```python
from build123d import *

# Parameters (mm, degrees)
SKETCH1_W                 = 3
SKETCH1_H                 = 15
BOSS_EXTRUDE1_START       = 9
SKETCH2_R                 = 5
BOSS_EXTRUDE1_DEPTH       = 9
M5X0_8_TAPPED_HOLE1_D     = 4.2
M5X0_8_TAPPED_HOLE1_DEPTH = 12.4
M5X0_8_TAPPED_HOLE1_TIP   = 1.2618073


with BuildPart() as part:
    # Sketch1 → Revolve1 (revolve)
    with BuildSketch(Plane.XY, mode=Mode.PRIVATE) as revolve1_sk:
        with Locations((-6.5, -4.132653061)):
            Rectangle(SKETCH1_W, SKETCH1_H)
    revolve(revolve1_sk.sketch.rotate(Axis((0, 8.367346939, 0), (0, -1, 0)), 270), axis=Axis((0, 8.367346939, 0), (0, -1, 0)))

    # Sketch2 → Boss-Extrude1 (add)
    with BuildSketch(Plane(origin=(0, 3.367346939, 0), x_dir=(1, 0, 0), z_dir=(0, 1, 0)).offset(BOSS_EXTRUDE1_START)):
        with BuildLine():
            Line((-6.5, 11.258330249), (-18.5, 4.330127019))
            ThreePointArc((-18.5, 4.330127019), (-21, 0), (-18.5, -4.330127019))
            Line((-18.5, -4.330127019), (-6.5, -11.258330249))
            ThreePointArc((-6.5, -11.258330249), (0, -13), (6.5, -11.258330249))
            Line((6.5, -11.258330249), (18.5, -4.330127019))
            ThreePointArc((18.5, -4.330127019), (21, 0), (18.5, 4.330127019))
            Line((18.5, 4.330127019), (6.5, 11.258330249))
            ThreePointArc((6.5, 11.258330249), (0, 13), (-6.5, 11.258330249))
        make_face()
        with Locations(Location((0, 0, 0), (0, 0, 270))):
            Circle(SKETCH2_R, mode=Mode.SUBTRACT)
    extrude(amount=-BOSS_EXTRUDE1_DEPTH)

    # M5x0.8 Tapped Hole1
    with Locations(Plane(origin=(-16, 12.367346939, 0), x_dir=(0, 0, 1), z_dir=(0, 1, 0))):
        with Locations((0, 0), (0, 32)):
            Hole(M5X0_8_TAPPED_HOLE1_D / 2, depth=M5X0_8_TAPPED_HOLE1_DEPTH)
            with Locations((0, 0, -(M5X0_8_TAPPED_HOLE1_DEPTH + M5X0_8_TAPPED_HOLE1_TIP / 2))):  # 118° drill point
                Cone(0, M5X0_8_TAPPED_HOLE1_D / 2, M5X0_8_TAPPED_HOLE1_TIP, mode=Mode.SUBTRACT)


solid = part.part
```
Geometry: final body of the model. Coordinates: model frame, mm. A direction names the side the tool comes from. Give positions to 0.01 mm unless a question says otherwise; leave off trailing zeros. Loops run counter-clockwise (first coordinate to the right, second up) from the corner with the lowest first, then second, coordinate; pieces in that order, holes last. Notation, with made-up numbers: (53.5, 5) -> (98.5, 5) arc R15 cw to (98.5, 12) -> close; hole circle Ø2 at (5.25, -10.5). An arc over 180 degrees is marked (long way). Return JSON: item names as keys, results as strings.
Item 1: Section B-B, the plane z = 0. Output: boundary loops of the cut face in (x, y).
Filled in:
{"outline": "(-21, 3.37) -> (-18.1, 3.37) -> (-18.1, 12.37) -> (-21, 12.37) -> close; (-13.9, 3.37) -> (-8, 3.37) -> (-8, -11.63) -> (-5, -11.63) -> (-5, 12.37) -> (-13.9, 12.37) -> close; (5, -11.63) -> (8, -11.63) -> (8, 3.37) -> (13.9, 3.37) -> (13.9, 12.37) -> (5, 12.37) -> close; (18.1, 3.37) -> (21, 3.37) -> (21, 12.37) -> (18.1, 12.37) -> close"}
Item 2: Section D-D, the plane z = -3.25. Output: boundary loops of the cut face in (x, y), plus the area to 3 significant figures.
Filled in:
{"outline": "(-19.8, 3.37) -> (-7.31, 3.37) -> (-7.31, -11.63) -> (-3.8, -11.63) -> (-3.8, 12.37) -> (-19.8, 12.37) -> close; (3.8, -11.63) -> (7.31, -11.63) -> (7.31, 3.37) -> (19.8, 3.37) -> (19.8, 12.37) -> (3.8, 12.37) -> close", "area": "393 mm^2"}
Item 3: Line query: line 1 (Z direction, x = 0, y = 6.25); line 2 (X direction, y = -7, z = 0); line 3 (Y direction, x = 12, z = 4). Output: solid intervals per line, ascending.
Filled in:
{"line 1": "-13 to -5, 5 to 13", "line 2": "-8 to -5, 5 to 8", "line 3": "3.37 to 12.37"}
Item 4: Mould query, pull axis X, two halves, no side actions, for faces 1 (the cylindrical face through (21, 8, 0)), 2 (the flat face through (5.2, -11.633, -0.1)), 3 (the cylindrical face through (17.77, 7.8, -1.13)), 4 (the cylindrical face through (-13.918, 7.804, 0.273)). Classes: released by +X, released by -X, zero draft, split by the parting line, or undercut.
Filled in:
{"face 1": "released by +X", "face 2": "zero draft", "face 3": "undercut", "face 4": "undercut"}
Item 5: Pin query (flat end, axial travel): P1, Ø10, axis at x = -16.5, y = 1.5, coming from the +Z side; P2, Ø3, axis at x = -6.5, y = 8.5, coming from the +Z side; P3, Ø6, axis at x = -6, y = 9.5, coming from the +Z side. Return the tip coordinate at first contact, or that it passes through.
Filled in:
{"P1": "z = 8.16", "P2": "z = 12", "P3": "z = 12.65"}
Item 6: Section A-A, the plane x = 0. Output: boundary loops of the cut face in (y, z).
Filled in:
{"outline": "(-11.63, -8) -> (3.37, -8) -> (3.37, -13) -> (12.37, -13) -> (12.37, -5) -> (-11.63, -5) -> close; (-11.63, 5) -> (12.37, 5) -> (12.37, 13) -> (3.37, 13) -> (3.37, 8) -> (-11.63, 8) -> close"}
Item 7: Access query for faces 5 (the cylindrical face through (0, 8, -13)), 6 (the flat face through (0, 3.367, -9)). Directions: +Z, -Z, +X, -X, +Y, -Y. A direction counts if a zero-diameter tool reaches every point of the face in a straight line with its end or side. Return the directions, or none.
Filled in:
{"face 5": "-Z, +Y, -Y", "face 6": "-Y"}
Item 8: Section C-C, the plane y = 6.25. Output: boundary loops of the cut face in (x, z), plus the area to 3 significant figures.
Filled in:
{"outline": "(-18.5, -4.33) -> (-6.5, -11.26) arc R13 ccw to (6.5, -11.26) -> (18.5, -4.33) arc R5 ccw to (18.5, 4.33) -> (6.5, 11.26) arc R13 ccw to (-6.5, 11.26) -> (-18.5, 4.33) arc R5 ccw to start; hole circle Ø4.2 at (-16, 0); hole circle Ø10 at (0, 0); hole circle Ø4.2 at (16, 0)", "area": "622 mm^2"}
